Design review of the part shown in the three views and the two pictorial views. Dimensions are in mm from the part's minimum x, y and z. A direction names the side the tool comes from. Give positions to 0.01 mm unless a question says otherwise; leave off trailing zeros. Loops run counter-clockwise (first coordinate to the right, second up) from the corner with the lowest first, then second, coordinate; pieces in that order, holes last. Notation, with made-up numbers: (81, 88) - (139, 88) arc R36 ccw to (139, 123) - close; hole circle Ø5 at (-22, 30). An arc over 180 degrees is marked (long way). Answer as a JSON object with one key per item and string values.
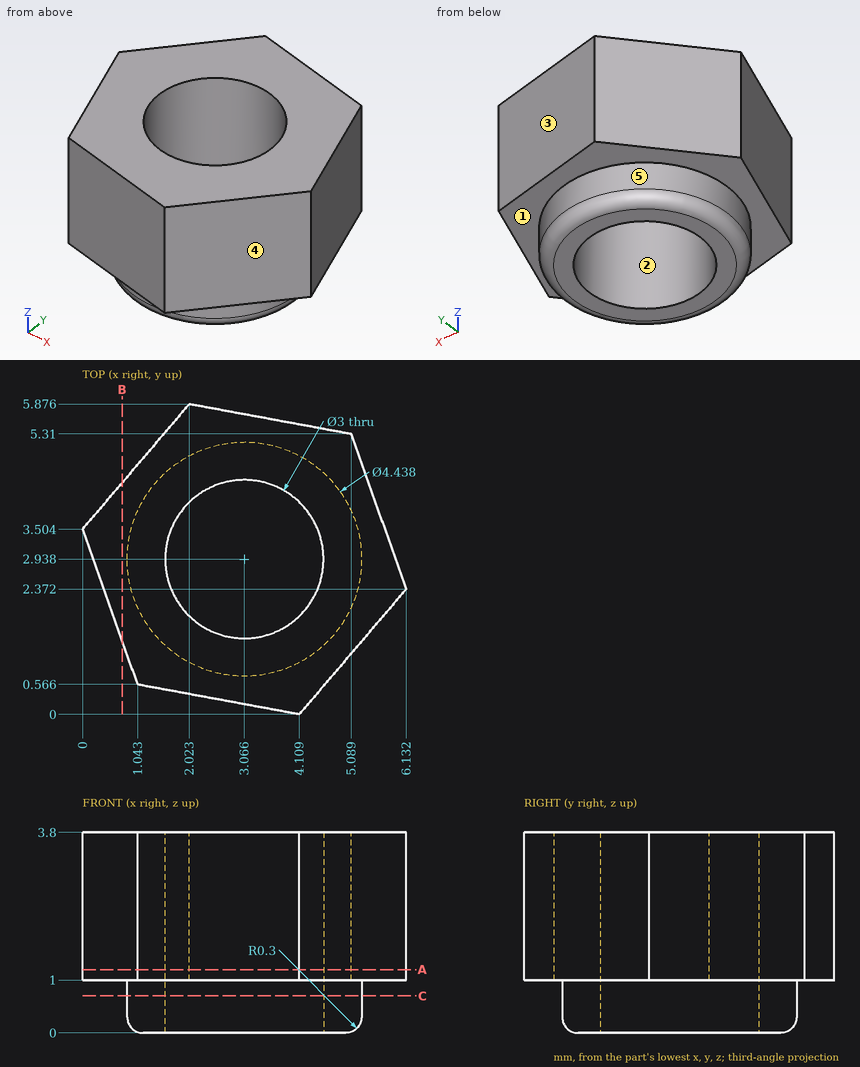
Q1. The part is to be moulded in two halves that separate along X. For the marked faces 1, 2 and 3, say which applies: +X half, -X half, draft (parallel to the pull), parting line (faces both ways), or undercut.
Results:
{"face 1": "draft", "face 2": "undercut", "face 3": "+X half"}
Q2. For the marked faces 4 and 5, list the 3-axis set-ups (+Z, -Z, +X, -X, +Y, -Y) from which the entire face can be reached by the end or side of a thin tool; tool diameter is ignored.
Results:
{"face 4": "+Z, -Z, +X, -Y", "face 5": "-Z"}
Q3. To check wall thickness, follow probe 1 along Z at (x, y) = (3.75, 0.6); probe 2 along X at (y, z) = (4.25, 0.8) (1 decimal); probe 3 along X at (y, z) = (2.85, 0.75). State the ranges of each line that lie inside material, in increasing order. Write a range as [from, to].
Results:
{"probe 1": "z = [1, 3.8]", "probe 2": "x = [1.3, 2.3], [3.8, 4.9]", "probe 3": "x = [0.85, 1.57], [4.56, 5.28]"}
Q4. Clearance check with flat-ended pins moving along their axes: pin 1 Ø2 at (x, z) = (2.5, 2.5) entering from +Y; pin 2 Ø1 at (x, z) = (3, 2) entering from -Y. State where each tip first meets the part, or that it passes through.
Results:
{"pin 1": "stops at y = 5.88", "pin 2": "stops at y = 0.11"}
Q5. Consider section A-A, the plane z = 1.2. State the section outline as (x, y) points (1 decimal), plus the area to 3 significant figures.
Results:
{"outline": "(0, 3.5) - (1, 0.6) - (4.1, 0) - (6.1, 2.4) - (5.1, 5.3) - (2, 5.9) - close; hole circle Ø3 at (3.1, 2.9)", "area": "18.2 mm^2"}
Q6. Consider section C-C, the plane z = 0.7. State the section outline as (x, y) points (1 decimal).
Results:
{"outline": "circle Ø4.4 at (3.1, 2.9); hole circle Ø3 at (3.1, 2.9)"}
Q7. Consider section B-B, the plane x = 0.75. State the section outline as (y, z) points.
Results:
{"outline": "(1.39, 1) - (4.38, 1) - (4.38, 3.8) - (1.39, 3.8) - close"}
